Design review of the part built by this model. Coordinates are the model's own, in mm. Face numbers are marked on the shaded views. A direction names the side the tool comes from. Give positions to 0.01 mm unless a question says otherwise; leave off trailing zeros. Loops run counter-clockwise (first coordinate to the right, second up) from the corner with the lowest first, then second, coordinate; pieces in that order, holes last. Notation, with made-up numbers: M 50.5,-15.75 L 58.5,-15.75 A12 cw 58.5,0.25 Z; hole C -24,-25.5 d1. An arc over 180 degrees is marked long. Use a Markdown table: item, result. Add a question column.
(1) Insertion check: pin 1 Ø12 at (y, z) = (13, 18.5) entering from +X; pin 2 Ø10 at (x, z) = (4.5, 20.5) entering from +Y; pin 3 Ø4.5 at (y, z) = (23.57, 23.57) entering from +X. Each pin has a flat end and moves straight along its axis. Give the tip position at first contact, or say it passes through.
(2) Add section D-D, the plane z = 0. Give the boundary of the cut face in (x, y) (3 decimals), then the cut area to 3 significant figures.
(3) For probe 1 along Y at (x, z) = (-38.5, 23.57); probe 2 along Z at (x, y) = (-53, -23); probe 3 along X at (y, z) = (-3.5, -11), list the stretches that pass through material, from the lowest coordinate up.
(4) Add section C-C, the plane x = -7.5. Give the boundary of the cut face in (y, z).
(5) Add section A-A, the plane y = 23.57. Give the boundary of the cut face in (x, z), then the cut area to 3 significant figures.
(6) For the marked faces 1 and 2, list the 3-axis set-ups (+Z, -Z, +X, -X, +Y, -Y) from which the entire face can be reached by the end or side of a thin tool; tool diameter is ignored.
```python
from build123d import *

# Parameters (mm, degrees)
SKETCH2_W           = 56.4
SKETCH2_H           = 56.4
BOSS_EXTRUDE1_DEPTH = 100
SKETCH3_R           = 2.5
CUT_EXTRUDE1_DEPTH  = 100
SKETCH4_R           = 3.175
BOSS_EXTRUDE2_DEPTH = 20.6


with BuildPart() as part:
    # Sketch2 → Boss-Extrude1 (new body)
    with BuildSketch(Plane(origin=(0, 0, 0), x_dir=(0, 0, -1), z_dir=(1, 0, 0))):
        Rectangle(SKETCH2_W, SKETCH2_H)
    extrude(amount=-BOSS_EXTRUDE1_DEPTH)

    # Sketch3 → Cut-Extrude1 (cut)
    with BuildSketch(Plane(origin=(0, 0, 0), x_dir=(0, 0, -1), z_dir=(1, 0, 0))):
        with Locations((-23.57, 23.57)):
            Circle(SKETCH3_R)
        with Locations(Location((23.57, 23.57, 0), (0, 0, 180))):
            Circle(SKETCH3_R)
        with Locations((23.57, -23.57)):
            Circle(SKETCH3_R)
        with Locations(Location((-23.57, -23.57, 0), (0, 0, 180))):
            Circle(SKETCH3_R)
    extrude(amount=-CUT_EXTRUDE1_DEPTH, mode=Mode.SUBTRACT)

    # Sketch4 → Boss-Extrude2 (add)
    with BuildSketch(Plane(origin=(0, 0, 0), x_dir=(0, 0, -1), z_dir=(1, 0, 0))):
        with Locations(Location((0, 0, 0), (0, 0, 180))):
            Circle(SKETCH4_R)
    extrude(amount=BOSS_EXTRUDE2_DEPTH)


solid = part.part
```
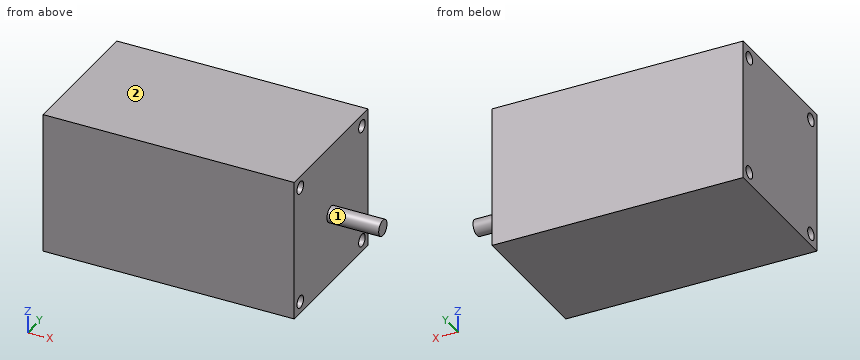
Established:
| question | item | result |
|---|---|---|
| 1 | pin 1 | x = 0 |
| 1 | pin 2 | y = 28.2 |
| 1 | pin 3 | through |
| 2 | outline | M -100,-28.2 L 0,-28.2 L 0,-3.175 L 20.6,-3.175 L 20.6,3.175 L 0,3.175 L 0,28.2 L -100,28.2 Z |
| 2 | area | 5,770 mm^2 |
| 3 | probe 1 | -28.2 to -26.07, -21.07 to 21.07, 26.07 to 28.2 |
| 3 | probe 2 | -28.2 to -26, -21.14 to 21.14, 26 to 28.2 |
| 3 | probe 3 | -100 to 0 |
| 4 | outline | M -28.2,-28.2 L 28.2,-28.2 L 28.2,28.2 L -28.2,28.2 Z; hole C -23.57,-23.57 d5; hole C -23.57,23.57 d5; hole C 23.57,-23.57 d5; hole C 23.57,23.57 d5 |
| 5 | outline | M -100,-28.2 L 0,-28.2 L 0,-26.07 L -100,-26.07 Z; M -100,-21.07 L 0,-21.07 L 0,21.07 L -100,21.07 Z; M -100,26.07 L 0,26.07 L 0,28.2 L -100,28.2 Z |
| 5 | area | 4,640 mm^2 |
| 6 | face 1 | +X |
| 6 | face 2 | +Z, +X, -X, +Y, -Y |
